Read the model definition and answer for the solid it produces. Units are mm, in the model's axes. Face numbers are marked on the shaded views. A direction names the side the tool comes from. Give positions to 0.01 mm unless a question says otherwise; leave off trailing zeros. Loops run counter-clockwise (first coordinate to the right, second up) from the corner with the lowest first, then second, coordinate; pieces in that order, holes last. Notation, with made-up numbers: (52.25, 17) - (78.25, 17) arc R26 cw to (78.25, 56) - close; hole circle Ø2 at (58, -16.5). An arc over 180 degrees is marked (long way). Put each result on its own line as item: value. Start each with the question number.
1. For the marked faces 4, 5 and 6, determine the directions among +Z, -Z, +X, -X, +Y, -Y from which every point of the face is accessible in a straight line to the end or side of a thin tool.
2. A cutting plane is placed at B-B, the plane x = 9.5. Count the separate pieces of the cut face and the enclosed holes in it, plus the area to 3 significant figures.
3. Given pin 1 Ø1.2 at (x, z) = (18, 6) entering from +Y; pin 2 Ø6 at (y, z) = (-2, 16.5) entering from +X; pin 3 Ø1 at (y, z) = (0.5, 7.5) entering from -X, each flat-ended and moving along its own axis, determine where each tip first touches the part or whether it passes through.
4. A cutting plane is placed at C-C, the plane z = 16.75. Determine the outline of the cut face in (x, y), plus the area to 3 significant figures.
5. For a pull along Y with two mould halves and no side action, classify the marked faces 1, 2 and 3 as released by +Y, released by -Y, zero draft, split by the parting line, or undercut.
6. A cutting plane is placed at A-A, the plane z = 4.5. Determine the outline of the cut face in (x, y).
7. Consider L1, parallel to Z at x = 13.2, y = 0; L2, parallel to X at y = 1, z = 7; L3, parallel to X at y = -1.75, z = 16.75. Determine where each line is inside the solid, lowest interval first. Write a range as from..to.
```python
from build123d import *

# Parameters (mm, degrees)
SKETCH_R        = 1.75
PAD_DEPTH       = 21
SKETCH002_W     = 5.5
SKETCH002_H     = 2.4
POCKET_DEPTH    = 8
SKETCH003_R     = 3.1
POCKET001_DEPTH = 3
SKETCH007_W     = 1.5
SKETCH007_H     = 2
SKETCH007_W_2   = 2.5
SKETCH007_H_2   = 1.5
POCKET002_DEPTH = 21.001
SKETCH008_W     = 10
SKETCH008_H     = 8
PAD001_DEPTH    = 10
CHAMFER_SIZE    = 4
SKETCH009_R     = 1.55
POCKET003_DEPTH = 13.001
POCKET004_DEPTH = 1
SKETCH011_W     = 10
SKETCH011_H     = 2
POCKET005_DEPTH = 7


with BuildPart() as part:
    # Sketch → Pad (new body)
    with BuildSketch(Plane.YZ):
        with BuildLine():
            Line((-5, 8), (-5, 10))
            Line((-5, 10), (5, 10))
            Line((5, 10), (5, 8))
            ThreePointArc((5, 8), (3.556624, 5.5), (5, 3))
            Line((5, 3), (5, 0))
            Line((5, 0), (2.5, 0))
            ThreePointArc((2.5, 0), (0, 1.443376), (-2.5, 0))
            Line((-2.5, 0), (-5, 0))
            Line((-5, 0), (-5, 3))
            ThreePointArc((-5, 3), (-3.556624, 5.5), (-5, 8))
        make_face()
        with Locations((0, 5)):
            Circle(SKETCH_R, mode=Mode.SUBTRACT)
    extrude(amount=PAD_DEPTH)

    # Sketch002 → Pocket (cut)
    with BuildSketch(Plane(origin=(0, 0, 10), x_dir=(0, -1, 0), z_dir=(0, 0, 1))):
        with Locations((0, 5.7)):
            Rectangle(SKETCH002_W, SKETCH002_H)
        with Locations((0, 18.2)):
            Rectangle(SKETCH002_W, SKETCH002_H)
    extrude(amount=-POCKET_DEPTH, mode=Mode.SUBTRACT)

    # Sketch003 (on Face4 of Pocket) → Pocket001 (cut)
    with BuildSketch(Plane(origin=(0, 0, 0), x_dir=(0, 1, 0), z_dir=(-1, 0, 0))):
        with Locations((0, -5)):
            Circle(SKETCH003_R)
    extrude(amount=-POCKET001_DEPTH, mode=Mode.SUBTRACT)

    # Sketch007 (on Face4 of Pocket001) → Pocket002 (cut, through all)
    with BuildSketch(Plane(origin=(0, 0, 0), x_dir=(0, 1, 0), z_dir=(-1, 0, 0))):
        with Locations((-3.5, -1.75)):
            Rectangle(SKETCH007_W, SKETCH007_H)
        with Locations((3.5, -1.75)):
            Rectangle(SKETCH007_W, SKETCH007_H)
        with Locations((-2.75, -8.75)):
            Rectangle(SKETCH007_W_2, SKETCH007_H_2)
        with Locations((2.75, -8.75)):
            Rectangle(SKETCH007_W_2, SKETCH007_H_2)
    extrude(amount=-POCKET002_DEPTH, mode=Mode.SUBTRACT)

    # Sketch008 (on Face3 of Pocket002) → Pad001 (join)
    with BuildSketch(Plane(origin=(0, 0, 10), x_dir=(0, -1, 0), z_dir=(0, 0, 1))):
        with Locations((0, 12)):
            Rectangle(SKETCH008_W, SKETCH008_H)
    extrude(amount=PAD001_DEPTH)

    # Chamfer
    chamfer_edges = [part.edges().sort_by_distance(p)[0] for p in [
        (12, -5, 20),
        (12, 5, 20),
    ]]
    chamfer(chamfer_edges, length=CHAMFER_SIZE)

    # Sketch009 (on Face5 of Chamfer) → Pocket003 (cut, through all)
    with BuildSketch(Plane(origin=(8, 0, 0), x_dir=(0, 1, 0), z_dir=(-1, 0, 0))):
        with Locations((0, -17)):
            Circle(SKETCH009_R)
    extrude(amount=-POCKET003_DEPTH, mode=Mode.SUBTRACT)

    # Sketch010 (on Face2 of Pocket003) → Pocket004 (cut)
    with BuildSketch(Plane.YZ.offset(16)):
        Polygon((3.175426, 17), (1.587713, 19.75), (-1.587713, 19.75), (-3.175426, 17), (-1.587713, 14.25), (1.587713, 14.25), align=None)
    extrude(amount=-POCKET004_DEPTH, mode=Mode.SUBTRACT)

    # Sketch011 (on Face17 of Pocket004) → Pocket005 (cut)
    with BuildSketch(Plane(origin=(0, 0, 20), x_dir=(0, -1, 0), z_dir=(0, 0, 1))):
        with Locations((0, 11.5)):
            Rectangle(SKETCH011_W, SKETCH011_H)
    extrude(amount=-POCKET005_DEPTH, mode=Mode.SUBTRACT)


solid = part.part
```
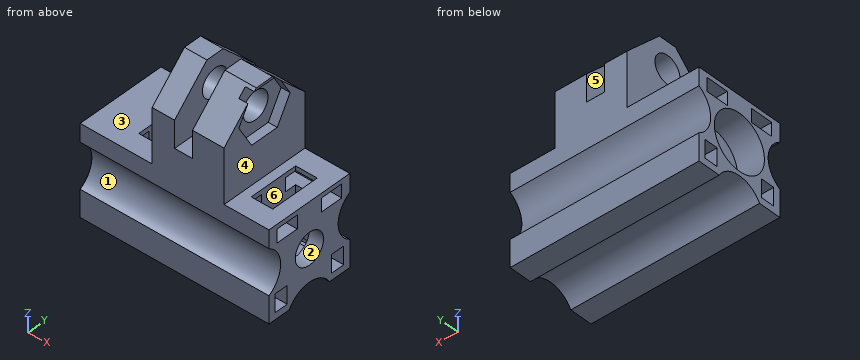
Return value:
1. face 4: +Z, +X, +Y, -Y
1. face 5: +Z, +Y, -Y
1. face 6: +Z
2. separate pieces: 1
2. enclosed holes: 6
2. area: 138 mm2
3. pin 1: stops at y = 3.77
3. pin 2: stops at x = 16
3. pin 3: stops at x = 3
4. outline: (8, -4.25) - (10.5, -4.25) - (10.5, -1.53) - (8, -1.53) - close; (8, 1.53) - (10.5, 1.53) - (10.5, 4.25) - (8, 4.25) - close; (12.5, -4.25) - (16, -4.25) - (16, -3.03) - (15, -3.03) - (15, -1.53) - (12.5, -1.53) - close; (12.5, 1.53) - (15, 1.53) - (15, 3.03) - (16, 3.03) - (16, 4.25) - (12.5, 4.25) - close
4. area: 29.6 mm2
5. face 1: released by -Y
5. face 2: undercut
5. face 3: zero draft
6. outline: (0, -3.74) - (21, -3.74) - (21, -1.68) - (19.4, -1.68) - (19.4, -2.75) - (17, -2.75) - (17, -1.68) - (6.9, -1.68) - (6.9, -2.75) - (4.5, -2.75) - (4.5, -1.68) - (3, -1.68) - (3, -3.06) - (0, -3.06) - close; (0, 3.06) - (3, 3.06) - (3, 1.68) - (4.5, 1.68) - (4.5, 2.75) - (6.9, 2.75) - (6.9, 1.68) - (17, 1.68) - (17, 2.75) - (19.4, 2.75) - (19.4, 1.68) - (21, 1.68) - (21, 3.74) - (0, 3.74) - close
7. L1: z = 1.44..3.25, 6.75..15.45, 18.55..20
7. L2: x = 3..4.5, 6.9..17, 19.4..21
7. L3: x = 8..10.5, 12.5..15
